from build123d import *

# Parameters (mm, degrees)
F0_R     = 7.9375
F1_DEPTH = 84.1375
F2_R     = 7.493
F3_DEPTH = 1.016
F4_R     = 7.9375
F5_DEPTH = 4.826
F6_SIZE  = 0.762


with BuildPart() as f1:
    # F0 (on Right) → F1 (new body, symmetric)
    with BuildSketch(Plane.YZ):
        Circle(F0_R)
    extrude(amount=F1_DEPTH, both=True)

    # F2 (on face) → F3 (join)
    with BuildSketch(Plane.YZ.offset(84.1375)):
        Circle(F2_R)
    extrude(amount=F3_DEPTH)

    # F4 (on face) → F5 (join)
    with BuildSketch(Plane.YZ.offset(85.1535)):
        Circle(F4_R)
    extrude(amount=F5_DEPTH)

    # F6
    f6_edges = [f1.edges().sort_by_distance(p)[0] for p in [
        (89.9795, -7.9375, 0),
    ]]
    chamfer(f6_edges, length=F6_SIZE)

    # F7: F1 across plane


with BuildPart() as f1_1:
    add(f1.part)
    add(f1.part.mirror(Plane.YZ))


solid = f1_1.part
Read the model definition and answer for the solid it produces. Units are mm, in the model's axes. A direction names the side the tool comes from. Coordinates: 2 decimals unless noted, no trailing zeros. Write each loop counter-clockwise with the first axis right and the second up, starting at its lowest first coordinate (ties: lowest second). Pieces come first, ordered by that corner, then holes. Notation, with made-up numbers: M -13.5,72 L 34.5,72 A28 ccw 34.5,108 Z; hole C 49,32 d3. An arc over 180 degrees is marked long. Use a Markdown table: item, result.
Q1. Which of the six approach directions +Z, -Z, +X, -X, +Y, -Y give full straight-line access (tool end or side, diameter ignored) to faces 5 (the face through (-87.16, -1.72, -7.75)), 6 (the face through (84.64, -0.98, 7.43))?
Answer block:
| item | result |
|---|---|
| face 5 | +X, -X |
| face 6 | none |
Q2. Determine the mould class of faces 1 (the face through (-84.64, -0.98, 7.43)), 2 (the face through (-89.979, 0, 0)), 3 (the face through (87.16, -1.72, -7.75)), 4 (the face through (89.979, 0, 0)) for opening direction X: released by +X, released by -X, zero draft, split by the parting line, or undercut.
Answer block:
| item | result |
|---|---|
| face 1 | undercut |
| face 2 | released by -X |
| face 3 | zero draft |
| face 4 | released by +X |
Q3. Each of these flat-tipped pins is pushed along its axis until it touches: pin 1 Ø6 at (x, z) = (46.5, -5) entering from -Y; pin 2 Ø2 at (x, y) = (55.5, -4) entering from +Z. Where does it stop, or does it pass through?
Answer block:
| item | result |
|---|---|
| pin 1 | stops at y = -7.68 |
| pin 2 | stops at z = 7.35 |
Q4. The part is cut by section A-A, the plane x = 72.5. Write down the section's boundary in (y, z) (1 decimal).
Answer block:
| item | result |
|---|---|
| outline | C 0,0 d15.9 |
Q5. Straight lines are drawn through the part: L1, parallel to Z at x = 22, y = -0.75; L2, parallel to X at y = -3.75, z = -6.75; L3, parallel to Y at x = 9, z = -0.5. For each, find the intervals that lie inside material, in ascending order. Write a range as [from, to].
Answer block:
| item | result |
|---|---|
| L1 | z = [-7.9, 7.9] |
| L2 | x = [-89.43, -85.15], [-84.14, 84.14], [85.15, 89.43] |
| L3 | y = [-7.92, 7.92] |
